Here's how the part is built. I have some questions about the finished solid (model axes, mm). A direction names the side the tool comes from. Round coordinates to 2 decimals unless told otherwise and drop trailing zeros. Loops run counter-clockwise (first coordinate to the right, second up) from the corner with the lowest first, then second, coordinate; pieces in that order, holes last. Notation, with made-up numbers: (26.5, 82) -> (57.5, 82) arc R14 cw to (57.5, 102) -> close; hole circle Ø2 at (-28, 47.25). An arc over 180 degrees is marked (long way). Use CSV: the item, a comma, the result in double quotes. Start each with the question number.
from build123d import *

# Parameters (mm, degrees)
SKETCH3_OUTSIDE_W  = 80
SKETCH3_OUTSIDE_H  = 80
CUT_EXTRUDE1_DEPTH = 31


with BuildPart() as part:
    # Sketch2 → Revolve1 (revolve)
    with BuildSketch(Plane.XY):
        Polygon((22.5, 0), (22.5, 17), (21, 17), (21, 20), (30, 20), (30, 30), (15, 30), (15, 29), (18, 25), (15, 25), (15, 16), (17, 16), (17, 13), (15, 13), (15, 8), (17, 8), (17, 5), (15, 5), (15, 0), align=None)
    revolve(axis=Axis((0, 16.306451613, 0), (0, -1, 0)))

    # Sketch3 outside → Cut-Extrude1 (cut, through all)
    with BuildSketch(Plane(origin=(0, 30, 0), x_dir=(1, 0, 0), z_dir=(0, 1, 0))):
        Rectangle(SKETCH3_OUTSIDE_W, SKETCH3_OUTSIDE_H)
        Polygon((0.936055849, 31.162859295), (-26.51979988, 16.392077792), (-27.455855728, -14.770781503), (-0.936055849, -31.162859295), (26.51979988, -16.392077792), (27.455855728, 14.770781503), align=None, mode=Mode.SUBTRACT)
    extrude(amount=-CUT_EXTRUDE1_DEPTH, mode=Mode.SUBTRACT)


solid = part.part
Q1. I want a section at A-A, the plane x = 20. List the corners of the cut face in (y, z) for me.
Q2. Will these pins go through, and if not, where does the flat tip stop? pin 1 Ø13.5 at (x, z) = (-1.5, 3.5) entering from +Y; pin 2 Ø10 at (y, z) = (5.5, -6.5) entering from +X; pin 3 Ø1 at (y, z) = (7.5, -21) entering from -X; pin 4 Ø6 at (y, z) = (4.5, -9.5) entering from -X.
Q3. I want a section at B-B, the plane z = 26.5. List the corners of the cut face in (x, y) for me, then the cut area to 3 significant figures.
Q4. I need wall thicknesses on line 1 along Z through (x, y) = (0, 14.1); line 2 along Z through (x, y) = (0, 3.65); line 3 along Y through (x, z) = (18, 20). Which ranges of each line are inside material? Lowest first, please.
Q5. For faces 4 (the flat face through (-15, 0, -5)), 5 (the flat face through (-6, 16, -14)), which set-ups out of +Z, -Z, +X, -X, +Y, -Y let a thin tool reach every point of the face, with its end or its side?
Q6. If we mould it in two halves opening along Z, with no side actions, what happens to faces 1 (the flat face through (-6, 8, -14)), 2 (the cylindrical face through (25.535, 25.07, 15.747)), 3 (the flat face through (20, 17, 7))? For each: pulls with the +Z half, pulls with the -Z half, needs draft (parallel to the pull), parting line crosses it, or undercut.
Values found:
1,outline,"(0, -10.31) -> (17, -10.31) -> (17, -6.4) -> (20, -6.4) -> (20, -19.38) -> (30, -19.38) -> (30, 19.9) -> (20, 19.9) -> (20, 6.4) -> (17, 6.4) -> (17, 10.31) -> (0, 10.31) -> close"
2,pin 1,"through"
2,pin 2,"x = 22.45"
2,pin 3,"x = -9.27"
2,pin 4,"x = -21.54"
3,outline,"(-8.48, 20) -> (7.73, 20) -> (7.73, 30) -> (-8.48, 30) -> close"
3,area,"162 mm2"
4,line 1,"-22.5 to -17, 17 to 22.5"
4,line 2,"-22.5 to -15, 15 to 22.5"
4,line 3,"20 to 30"
5,face 4,"+Z, -Z, +X, -X, -Y"
5,face 5,"none"
6,face 1,"undercut"
6,face 2,"pulls with the +Z half"
6,face 3,"needs draft"
